```python
from build123d import *

# Parameters (mm, degrees)
F1_DEPTH  = 12.7
F2_W      = 17.557748
F2_H      = 3.1115
F3_DEPTH  = 2.54
F5_DEPTH  = 2.54
F6_W      = 5.349429
F6_H      = 5.349428
F7_DEPTH  = 2.54
F8_R      = 2.389631
F9_DEPTH  = 2.54
F10_R     = 2.235372
F11_DEPTH = 12.7


with BuildPart() as f1:
    # F0 (on Front) → F1 (new body)
    with BuildSketch(Plane.XZ):
        Polygon((-14.136652, 29.049095), (-14.136652, 0), (-14.136652, -15.400905), (11.263348, -15.400905), (11.263348, 29.049095), align=None)
    extrude(amount=F1_DEPTH)

    # F2 (on face) → F3 (cut)
    with BuildSketch(Plane.XZ.offset(12.7)):
        with Locations((-1.666876, 22.447251)):
            Rectangle(F2_W, F2_H)
    extrude(amount=-F3_DEPTH, mode=Mode.SUBTRACT)

    # F4 (on face) → F5 (join)
    with BuildSketch(Plane.XZ.offset(12.7)):
        Polygon((2.2225, 5.11175), (-3.77825, 8.223251), (-3.77825, 3.1115), align=None)
    extrude(amount=F5_DEPTH)

    # F6 (on face) → F7 (join)
    with BuildSketch(Plane.XZ.offset(12.7)):
        with Locations((-10.126119, 5.396833)):
            Rectangle(F6_W, F6_H)
    extrude(amount=F7_DEPTH)

    # F8 (on face) → F9 (join)
    with BuildSketch(Plane.XZ.offset(12.7)):
        with Locations((6.446437, 5.11175)):
            Circle(F8_R)
    extrude(amount=F9_DEPTH)

    # F10 (on face) → F11 (cut)
    with BuildSketch(Plane(origin=(0, 0, -15.400905), x_dir=(1, 0, 0), z_dir=(0, 0, -1))):
        with Locations((-8.754111, 6.379303)):
            Circle(F10_R)
    extrude(amount=-F11_DEPTH, mode=Mode.SUBTRACT)


solid = f1.part
```
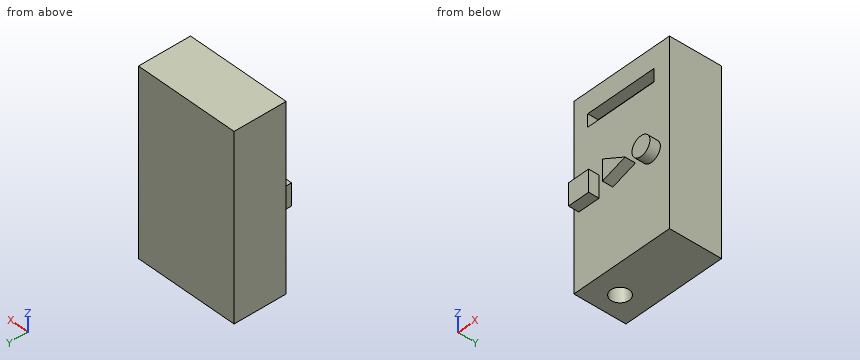
Verification items for the finished model (mm, model axes). Coordinates: 2 decimals unless noted, no trailing zeros. Loops run counter-clockwise (first coordinate to the right, second up) from the corner with the lowest first, then second, coordinate; pieces in that order, holes last. Notation, with made-up numbers: (49.5, 86.25) -> (60.5, 86.25) arc R23 ccw to (60.5, 119.25) -> close; hole circle Ø3 at (29.5, 35). An arc over 180 degrees is marked (long way). Answer in a Markdown table with one row per item. Add a question column.
1. Section check A-A, the plane x = -12. Enter the section's corners in (y, z), then the cut area to 3 significant figures.
2. Section check D-D, the plane x = 6.25. Enter the section's corners in (y, z), then the cut area to 3 significant figures.
3. Material ranges on probe 1 along Z at (x, y) = (-3.5, -12.5); probe 2 along X at (y, z) = (-10.25, 21.5); probe 3 along Y at (x, z) = (7.5, -6), recorded low to high. Write a range as [from, to].
4. Depth check by flat-ended pin: P1, Ø2.5, axis at x = 0.5, z = 23, coming from the -Y side; P2, Ø2, axis at x = -10, y = -14, coming from the -Z side; P3, Ø1.3, axis at y = -13.5, z = 6.5, coming from the -X side. Enter the tip coordinate at first touch or a pass-through.
5. Section check C-C, the plane z = -9. Enter the section's corners in (x, y).
6. Section check B-B, the plane y = -4.75. Enter the section's corners in (x, z).
Derived:
| question | item | result |
|---|---|---|
| 1 | outline | (-15.24, 2.72) -> (-12.7, 2.72) -> (-12.7, -15.4) -> (0, -15.4) -> (0, 29.05) -> (-12.7, 29.05) -> (-12.7, 8.07) -> (-15.24, 8.07) -> close |
| 1 | area | 578 mm² |
| 2 | outline | (-15.24, 2.73) -> (-12.7, 2.73) -> (-12.7, -15.4) -> (0, -15.4) -> (0, 29.05) -> (-12.7, 29.05) -> (-12.7, 24) -> (-10.16, 24) -> (-10.16, 20.89) -> (-12.7, 20.89) -> (-12.7, 7.49) -> (-15.24, 7.49) -> close |
| 2 | area | 569 mm² |
| 3 | probe 1 | z = [-15.4, 20.89], [24, 29.05] |
| 3 | probe 2 | x = [-14.14, -10.45], [7.11, 11.26] |
| 3 | probe 3 | y = [-12.7, 0] |
| 4 | P1 | stops at y = -12.7 |
| 4 | P2 | stops at z = 2.72 |
| 4 | P3 | stops at x = -12.8 |
| 5 | outline | (-14.14, -12.7) -> (11.26, -12.7) -> (11.26, 0) -> (-14.14, 0) -> close; hole circle Ø4.47 at (-8.75, -6.38) |
| 6 | outline | (-14.14, -15.4) -> (-10.28, -15.4) -> (-10.28, -2.7) -> (-7.22, -2.7) -> (-7.22, -15.4) -> (11.26, -15.4) -> (11.26, 29.05) -> (-14.14, 29.05) -> close |
